```python
from build123d import *

# Parameters (mm, degrees)
BOSS_EXTRUDE1_START = 5
SKETCH2_W           = 63.507
SKETCH2_H           = 52.644
BOSS_EXTRUDE1_DEPTH = 2
SKETCH5_W           = 4.5
SKETCH5_H           = 3.844091241
BOSS_EXTRUDE2_DEPTH = 52.5
SKETCH8_W           = 3.84
SKETCH8_H           = 4.5
CUT_EXTRUDE1_DEPTH  = 5
SKETCH9_W           = 3.844091241
SKETCH9_H           = 4.5
CUT_EXTRUDE2_DEPTH  = 5
FILLET1_R           = 1
BOSS_EXTRUDE3_START = -2
SKETCH10_W          = 3.844091241
SKETCH10_H          = 8.427653373
BOSS_EXTRUDE3_DEPTH = 2.5
FILLET2_R           = 5
SKETCH11_R          = 1.25
CUT_EXTRUDE3_DEPTH  = 5
CUT_EXTRUDE4_START  = -5
SKETCH12_R          = 1.25
CUT_EXTRUDE4_DEPTH  = 5
SKETCH16_R          = 1.26021762
CUT_EXTRUDE5_DEPTH  = 4


with BuildPart() as part:
    # Sketch2 → Boss-Extrude1 (new body)
    with BuildSketch(Plane.XY.offset(20).offset(BOSS_EXTRUDE1_START)):
        with Locations((89.8185, 54.102)):
            Rectangle(SKETCH2_W, SKETCH2_H)
    extrude(amount=BOSS_EXTRUDE1_DEPTH)

    # Sketch5 → Boss-Extrude2 (add)
    with BuildSketch(Plane.XZ.offset(-27.78)):
        with Locations((60.315, 23.077954379)):
            Rectangle(SKETCH5_W, SKETCH5_H)
    extrude(amount=-BOSS_EXTRUDE2_DEPTH)

    # Sketch8 → Cut-Extrude1 (cut)
    with BuildSketch(Plane.ZY.offset(-58.065)):
        with Locations((23.075908759, 30.03)):
            Rectangle(SKETCH8_W, SKETCH8_H)
    extrude(amount=-CUT_EXTRUDE1_DEPTH, mode=Mode.SUBTRACT)

    # Sketch9 → Cut-Extrude2 (cut)
    with BuildSketch(Plane.ZY.offset(-58.065)):
        with Locations((23.077954379, 78.174)):
            Rectangle(SKETCH9_W, SKETCH9_H)
    extrude(amount=-CUT_EXTRUDE2_DEPTH, mode=Mode.SUBTRACT)

    # Fillet1
    fillet1_edges = [part.edges().sort_by_distance(p)[0] for p in [
        (58.065, 54.102, 21.155908759),
        (62.565, 54.102, 21.155908759),
    ]]
    fillet(fillet1_edges, radius=FILLET1_R)

    # Sketch10 → Boss-Extrude3 (add)
    with BuildSketch(Plane(origin=(121.572, 0, 0), x_dir=(0, 0, -1), z_dir=(1, 0, 0)).offset(BOSS_EXTRUDE3_START)):
        with Locations((-23.077954379, 52.638173314)):
            Rectangle(SKETCH10_W, SKETCH10_H)
    extrude(amount=-BOSS_EXTRUDE3_DEPTH)

    # Fillet2
    # the kernel refuses this fillet: 5 mm, written as the material it takes off along each edge
    with BuildSketch(Plane(origin=(131.733382256, 56.852, 21.155908759), x_dir=(0, 0, 1), z_dir=(-1, 0, 0))) as fillet2_piece_1:
        with BuildLine():
            CenterArc((5, -4.864552903), FILLET2_R, 103.366656392, 76.633343608)
            Line((0, -4.864552903), (-0.1, -4.864552903))
            Line((-0.1, -4.864552903), (-0.1, 0))
            Line((-0.1, 0), (0, 0.1))
            ThreePointArc((0, 0.1), (1.922045621, 0.1), (3.820973066, 0.097291058))
            Line((3.820973066, 0.097291058), (3.844091241, 0))
        make_face()
    extrude(amount=26.822764513, mode=Mode.SUBTRACT)
    with BuildSketch(Plane(origin=(131.733382256, 48.424346627, 21.155908759), x_dir=(0, 0, 1), z_dir=(-1, 0, 0))) as fillet2_piece_2:
        with BuildLine():
            CenterArc((5, 4.864552903), FILLET2_R, 180, 76.633343608)
            Line((0, 4.864552903), (-0.1, 4.864552903))
            Line((-0.1, 4.864552903), (-0.1, 0))
            Line((-0.1, 0), (0, -0.1))
            ThreePointArc((0, -0.1), (1.922045621, -0.1), (3.820973066, -0.097291058))
            Line((3.820973066, -0.097291058), (3.844091241, 0))
        make_face()
    extrude(amount=26.822764513, mode=Mode.SUBTRACT)

    # Sketch11 → Cut-Extrude3 (cut)
    with BuildSketch(Plane(origin=(0, 32.28, 0), x_dir=(-1, 0, 0), z_dir=(0, -1, 0))):
        with Locations(Location((-60.565, -23.295908759, 0), (0, 0, 90))):
            Circle(SKETCH11_R)
    extrude(amount=-CUT_EXTRUDE3_DEPTH, mode=Mode.SUBTRACT)

    # Sketch12 → Cut-Extrude4 (cut)
    with BuildSketch(Plane(origin=(0, 75.924, 0), x_dir=(1, 0, 0), z_dir=(0, 1, 0)).offset(CUT_EXTRUDE4_START)):
        with Locations(Location((60.565, -23.295908759, 0), (0, 0, 90))):
            Circle(SKETCH12_R)
    extrude(amount=CUT_EXTRUDE4_DEPTH, mode=Mode.SUBTRACT)

    # Sketch16 → Cut-Extrude5 (cut)
    with BuildSketch(Plane(origin=(119.572, 0, 0), x_dir=(0, 0, -1), z_dir=(1, 0, 0))):
        with Locations((-23.10766013, 52.666921641)):
            Circle(SKETCH16_R)
    extrude(amount=-CUT_EXTRUDE5_DEPTH, mode=Mode.SUBTRACT)


solid = part.part
```
CAD build for the part. Positions are in the model's coordinates, mm. A direction names the side the tool comes from. Round coordinates to 2 decimals unless told otherwise and drop trailing zeros. Order: outer loops, then holes, each group sorted by start corner. A loop starts at its lowest first (then second) coordinate and runs counter-clockwise, first axis right, second up. Notation, with made-up numbers: (-9.5, -18.5) - (1.5, -18.5) arc R16 cw to (1.5, 2.5) - close; hole circle Ø2 at (54, 1). An arc over 180 degrees is marked (long way). Answer as CSV lines item,"result". Start each with the question number.
1. Pull direction X, two halves, no side cores. Call faces 1 (the face through (61, 70.924, 23)), 2 (the face through (58.065, 54, 25)), 3 (the face through (118.3, 55.4, 22.5)), 4 (the face through (121.572, 54, 26)): +X half, -X half, draft (parallel to the pull), parting line (faces both ways), or undercut.
2. Drill centre lines: L1, parallel to X at y = 58.5, z = 23.65 (3 decimals); L2, parallel to X at y = 49.5, z = 23.25 (3 decimals); L3, parallel to Z at x = 113.5, y = 68.5. Where is each one in solid material? Low to high. Write a range as [from, to].
3. Saw through at B-B, the plane y = 59.5. Write the cut outline in (x, z) (3 decimals), and give its area (3 significant figures).
4. Saw through at C-C, the plane y = 73. Write the cut outline in (x, z) (3 decimals), and give its area (3 significant figures).
5. Pin check, flat tips, straight feed: pin 1 (1.1 mm diameter, centred on y = 52.5, z = 24, fed in from +X); pin 2 (4 mm diameter, centred on x = 89.5, y = 59.5, fed in from -Z); pin 3 (1.2 mm diameter, centred on x = 61, z = 23, fed in from +Y). Stop position of each tip, or through.
6. Tool access for faces 5 (the face through (118.34, 49.971, 22.415)), 6 (the face through (117.072, 54, 24)), 7 (the face through (59.456, 34.745, 22.719)), 8 (the face through (118.34, 52.722, 24.367)), 9 (the face through (59, 75.924, 23)): list every direction of +Z, -Z, +X, -X, +Y, -Y with a clear straight run to the whole face (end or side of a thin tool).
7. Saw through at D-D, the plane x = 70.5. Write the cut outline in (y, z).
8. Saw through at A-A, the plane z = 23.7. Write the cut outline in (x, y) (3 decimals).
Model answer:
1,face 1,"undercut"
1,face 2,"-X half"
1,face 3,"draft"
1,face 4,"+X half"
2,L1,"x = [58.065, 62.565]"
2,L2,"x = [58.065, 62.565], [117.072, 119.572]"
2,L3,"z = [25, 27]"
3,outline,"(58.065, 22.156) arc R1 ccw to (59.065, 21.156) - (61.565, 21.156) arc R1 ccw to (62.565, 22.156) - (62.565, 25) - (121.572, 25) - (121.572, 27) - (58.065, 27) - close"
3,area,"144 mm²"
4,outline,"(58.065, 22.156) arc R1 ccw to (59.065, 21.156) - (61.565, 21.156) arc R1 ccw to (62.565, 22.156) - (62.565, 25) - (121.572, 25) - (121.572, 27) - (58.065, 27) - close; hole circle Ø2.5 at (60.565, 23.296)"
4,area,"139 mm²"
5,pin 1,"stops at x = 119.57"
5,pin 2,"stops at z = 25"
5,pin 3,"stops at y = 70.92"
6,face 5,"-Z, +X, -Y"
6,face 6,"-Z, +Y, -Y"
6,face 7,"-Y"
6,face 8,"+X"
6,face 9,"-Z, +X, -X, +Y"
7,outline,"(27.78, 25) - (80.42, 25) - (80.42, 27) - (27.78, 27) - close"
8,outline,"(58.065, 32.28) - (59.382, 32.28) - (59.382, 37.28) - (61.748, 37.28) - (61.748, 32.28) - (62.565, 32.28) - (62.565, 75.924) - (61.748, 75.924) - (61.748, 70.924) - (59.382, 70.924) - (59.382, 75.924) - (58.065, 75.924) - close; (117.072, 48.934) - (119.572, 48.934) - (119.572, 51.555) - (117.072, 51.555) - close; (117.072, 53.779) - (119.572, 53.779) - (119.572, 56.343) - (117.072, 56.343) - close"
